from build123d import *

# Parameters (mm, degrees)
F0_W     = 127
F0_H     = 101.6
F1_DEPTH = 25.4
F2_DEPTH = 6.35
F3_T     = -2.54
F4_R     = 5.08


with BuildPart() as f1:
    # F0 (on Right) → F1 (new body)
    with BuildSketch(Plane.YZ):
        with Locations((63.5, 50.8)):
            Rectangle(F0_W, F0_H)
    extrude(amount=F1_DEPTH)

    # F0 (on Right) → F2 (join)
    with BuildSketch(Plane.YZ):
        with Locations((63.5, 50.8)):
            Rectangle(F0_W, F0_H)
    extrude(amount=F2_DEPTH)

    # F3
    f3_openings = [f1.faces().sort_by_distance(p)[0] for p in [
        (25.4, 63.5, 50.8),
    ]]
    offset(amount=F3_T, openings=f3_openings)

    # F4
    f4_edges = [f1.edges().sort_by_distance(p)[0] for p in [
        (12.7, 0, 101.6),
        (12.7, 0, 0),
        (12.7, 127, 0),
        (12.7, 127, 101.6),
    ]]
    fillet(f4_edges, radius=F4_R)


solid = f1.part
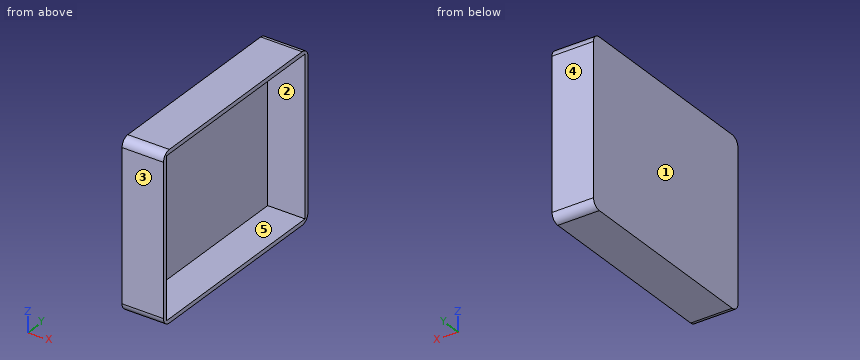
Verification items for the finished model (mm, model axes). Face numbers are marked on the shaded views. A direction names the side the tool comes from. Coordinates: 2 decimals unless noted, no trailing zeros. Loops run counter-clockwise (first coordinate to the right, second up) from the corner with the lowest first, then second, coordinate; pieces in that order, holes last. Notation, with made-up numbers: M 74,-9.75 L 112,-9.75 A10 cw 112,-2.75 Z; hole C 29,85.5 d6. An arc over 180 degrees is marked long. One line per item, written item: value.
1. Set-up check for the marked faces 1 and 2: record each of +Z, -Z, +X, -X, +Y, -Y from which the full face is reachable in a straight line by a thin tool's end or side.
Answers follow:
face 1: +Z, -Z, -X, +Y, -Y
face 2: +X
2. Gauge pin test, flat end, axial feed: P1, Ø5, axis at y = 68, z = 25.5, coming from the +X side. Record the tip position at first contact, or that the pin passes through.
Answers follow:
P1: x = 2.54
3. Section check C-C on y = 110. Record the cut outline in (x, z).
Answers follow:
outline: M 0,0 L 25.4,0 L 25.4,2.54 L 2.54,2.54 L 2.54,99.06 L 25.4,99.06 L 25.4,101.6 L 0,101.6 Z
4. Mould release check, pull along Y, two halves, no side actions. Record for the marked faces 3, 4 and 5: pulls with the +Y half, pulls with the -Y half, needs draft (parallel to the pull), parting line crosses it, or undercut.
Answers follow:
face 3: pulls with the -Y half
face 4: pulls with the +Y half
face 5: undercut
5. Section check B-B on z = 16.5. Record the cut outline in (x, y).
Answers follow:
outline: M 0,0 L 25.4,0 L 25.4,2.54 L 2.54,2.54 L 2.54,124.46 L 25.4,124.46 L 25.4,127 L 0,127 Z
6. Section check A-A on x = 9. Record the cut outline in (y, z).
Answers follow:
outline: M 0,5.08 A5.08 ccw 5.08,0 L 121.92,0 A5.08 ccw 127,5.08 L 127,96.52 A5.08 ccw 121.92,101.6 L 5.08,101.6 A5.08 ccw 0,96.52 Z; hole M 2.54,2.54 L 124.46,2.54 L 124.46,99.06 L 2.54,99.06 Z
7. Material ranges on line 1 along Z through (x, y) = (21, 19); line 2 along Y through (x, z) = (23.25, 41); line 3 along X through (y, z) = (20.5, 85), recorded low to high. Write a range as from..to.
Answers follow:
line 1: 0..2.54, 99.06..101.6
line 2: 0..2.54, 124.46..127
line 3: 0..2.54
